Can you work these out from the drawing? Everything is in mm from the part's minimum corner. Coordinates: 2 decimals unless noted, no trailing zeros. Loops run counter-clockwise (first coordinate to the right, second up) from the corner with the lowest first, then second, coordinate; pieces in that order, holes last. Notation, with made-up numbers: (-37, 16) - (8, 16) arc R15 ccw to (8, 29) - close; hole circle Ø7 at (41.5, 38). An arc over 180 degrees is marked (long way). Put each result on its own line as item: value. Start each with the question number.
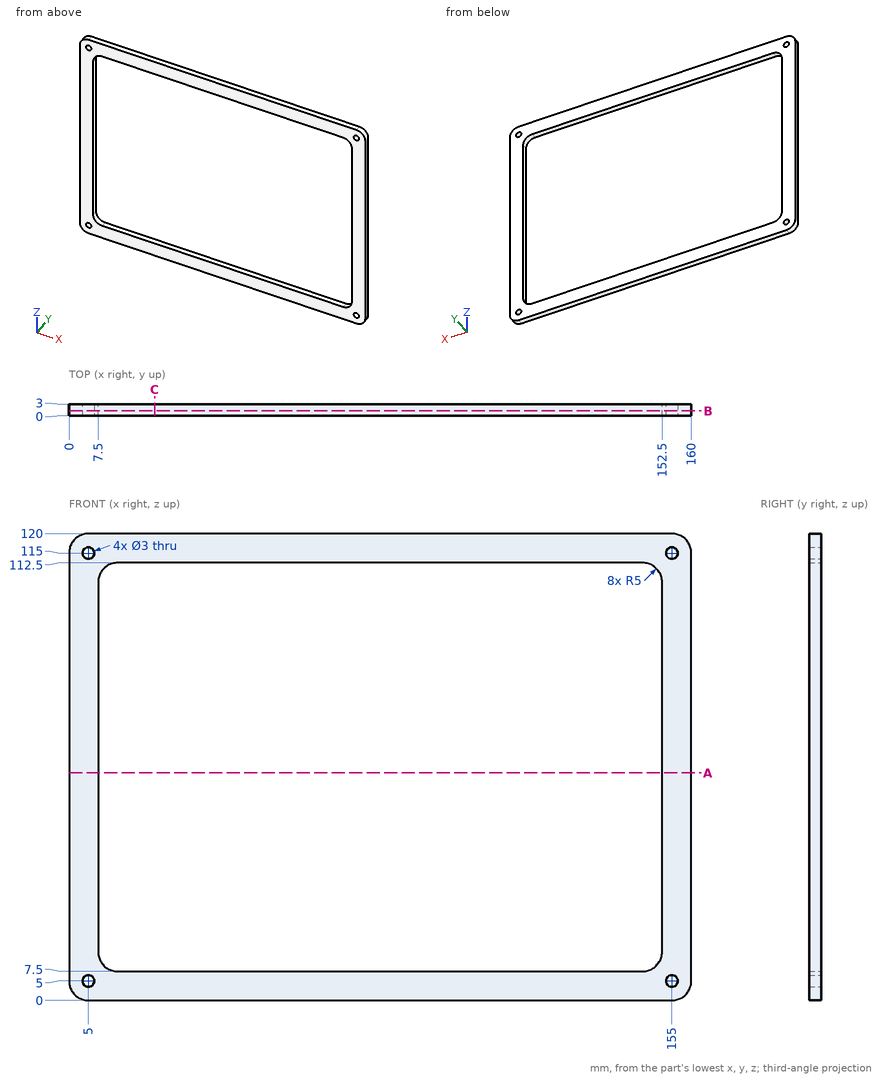
Q1. I want a section at A-A on z = 58.5. List the corners of the cut face in (x, y) for me, and give its area (3 significant figures).
Q2. I want a section at B-B on y = 1.25. List the corners of the cut face in (x, z) for me.
Q3. I want a section at C-C on x = 22. List the corners of the cut face in (y, z) for me.
Q4. Please list where these lines run through material, in increasing order: line 1 along Z through (x, y) = (155, 0.8); line 2 along X through (y, z) = (0.85, 26); line 3 along Z through (x, y) = (22, 0.15). Write a range as [from, to].
Calculated:
1. outline: (0, 0) - (7.5, 0) - (7.5, 3) - (0, 3) - close; (152.5, 0) - (160, 0) - (160, 3) - (152.5, 3) - close
1. area: 45.0 mm2
2. outline: (0, 5) arc R5 ccw to (5, 0) - (155, 0) arc R5 ccw to (160, 5) - (160, 115) arc R5 ccw to (155, 120) - (5, 120) arc R5 ccw to (0, 115) - close; hole circle Ø3 at (5, 5); hole circle Ø3 at (5, 115); hole (7.5, 12.5) arc R5 ccw to (12.5, 7.5) - (147.5, 7.5) arc R5 ccw to (152.5, 12.5) - (152.5, 107.5) arc R5 ccw to (147.5, 112.5) - (12.5, 112.5) arc R5 ccw to (7.5, 107.5) - close; hole circle Ø3 at (155, 5); hole circle Ø3 at (155, 115)
3. outline: (0, 0) - (3, 0) - (3, 7.5) - (0, 7.5) - close; (0, 112.5) - (3, 112.5) - (3, 120) - (0, 120) - close
4. line 1: [0, 3.5], [6.5, 113.5], [116.5, 120]
4. line 2: [0, 7.5], [152.5, 160]
4. line 3: [0, 7.5], [112.5, 120]
